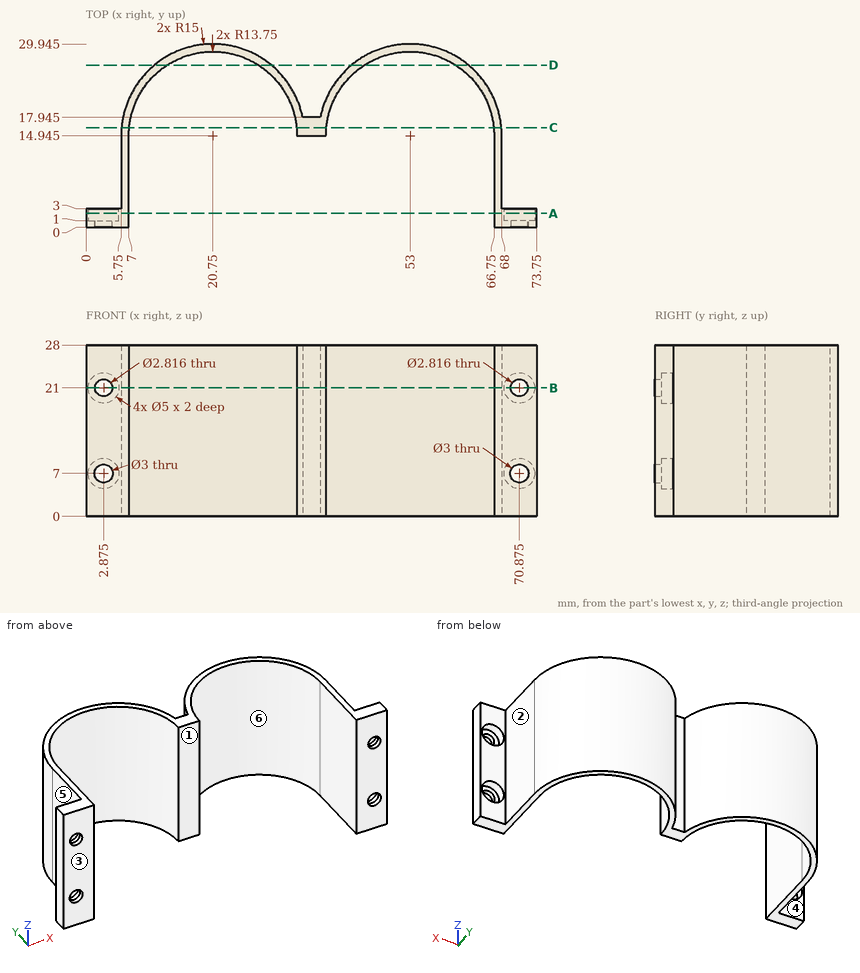
Can you work these out from the drawing? Everything is in mm from the part's minimum corner. A direction names the side the tool comes from. Coordinates: 2 decimals unless noted, no trailing zeros. Loops run counter-clockwise (first coordinate to the right, second up) from the corner with the lowest first, then second, coordinate; pieces in that order, holes last. Notation, with made-up numbers: (-17.75, 28) - (-7.75, 28) arc R32 cw to (-7.75, 64) - close; hole circle Ø9 at (35.25, 3). An arc over 180 degrees is marked (long way). Put each result on its own line as item: value. Start each with the question number.
Item 1: Suppose I cut it at B-B (z = 21). State how many separate pieces and enclosed holes the cut face has.
Item 2: Suppose I cut it at D-D (y = 26.5). Please give me the cut outline in (x, z) (1 decimal).
Item 3: If we mould it in two halves opening along X, with no side actions, what happens to the marked faces 4, 5 and 6? For each: +X half, -X half, draft (parallel to the pull), parting line (faces both ways), or undercut.
Item 4: For pin 1 (6 mm diameter, centred on x = 2.875, z = 21, fed in from -Y); pin 2 (1.5 mm diameter, centred on y = 25.5, z = 16, fed in from +X); pin 3 (4.5 mm diameter, centred on x = 2.875, z = 7, fed in from +Y); pin 4 (5 mm diameter, centred on x = 54, z = 23, fed in from -Y), each with a flat end and sliding along its axis, tell me the tip position at first contact or that it passes through.
Item 5: Suppose I cut it at A-A (y = 2.25). Please give me the cut outline in (x, z) (3 decimals).
Item 6: Which directions (+Z, -Z, +X, -X, +Y, -Y) give clear straight access to the entire face, cutting with the end or side of a thin tool? Please do the marked faces 1, 2 and 3.
Item 7: Suppose I cut it at C-C (y = 16.25). Please give me the cut outline in (x, z).
Item 8: If I drill on line 1 along X through (y, z) = (3.75, 25.5); line 2 along Y through (x, z) = (37.5, 15.5) (1 decimal); line 3 along Y through (x, z) = (68.5, 12.25), over which ranges is the centre line in solid material (lowest first)?
Here are the results:
1. separate pieces: 3
1. enclosed holes: 0
2. outline: (11.2, 0) - (13.3, 0) - (13.3, 28) - (11.2, 28) - close; (28.2, 0) - (30.3, 0) - (30.3, 28) - (28.2, 28) - close; (43.4, 0) - (45.5, 0) - (45.5, 28) - (43.4, 28) - close; (60.5, 0) - (62.6, 0) - (62.6, 28) - (60.5, 28) - close
3. face 4: draft
3. face 5: -X half
3. face 6: undercut
4. pin 1: y = 0
4. pin 2: x = 64.35
4. pin 3: y = 1
4. pin 4: y = 28.24
5. outline: (0, 0) - (7, 0) - (7, 28) - (0, 28) - close; (66.75, 0) - (73.75, 0) - (73.75, 28) - (66.75, 28) - close; hole circle Ø5 at (2.875, 7); hole circle Ø5 at (2.875, 21); hole circle Ø5 at (70.875, 7); hole circle Ø5 at (70.875, 21)
6. face 1: +Z, -Z, -Y
6. face 2: +Z, -Z, +X, +Y
6. face 3: +Z, -Z, +X, -X, -Y
7. outline: (5.81, 0) - (7.06, 0) - (7.06, 28) - (5.81, 28) - close; (34.44, 0) - (39.31, 0) - (39.31, 28) - (34.44, 28) - close; (66.69, 0) - (67.94, 0) - (67.94, 28) - (66.69, 28) - close
8. line 1: 5.75 to 7, 66.75 to 68
8. line 2: 14.9 to 17.9
8. line 3: 0 to 3
